Autodesk Inventor part; units mm, degrees
ref_plane "Start Plane" through (0, 0, -14.2929) normal (0, 0, 1) x (1, 0, 0)
ref_plane "End Plane" through (0, 0, 514.2929) normal (0, 0, 1) x (1, 0, 0)
ref_plane "Work Plane11" through (-7.7636, 7.7, -14.6464) normal (0.7071, 0, -0.7071) x (-0.7071, 0, -0.7071)
ref_plane "Start Plane" through (0, 0, -14.2929) normal (0, 0, 1) x (1, 0, 0)
ref_plane "End Plane" through (0, 0, 514.2929) normal (0, 0, 1) x (1, 0, 0)
sketch "Sketch" plane through (0, 0, 0) normal (0, 0, 1) x (1, 0, 0)
  line L0 (-2.41, 28.7) -> (-2.41, -7.3)
  line L1 (-7.41, 32.7) -> (-6.41, 32.7)
  line L2 (-7.41, -17.3) -> (-7.41, 32.7)
  line L3 (22.59, -17.3) -> (-7.41, -17.3)
  line L4 (22.59, -16.3) -> (22.59, -17.3)
  line L5 (2.59, -12.3) -> (18.59, -12.3)
  arc A0 (-2.41, -7.3) -> (2.59, -12.3) centre (2.59, -7.3) ccw
  arc A1 (-2.41, 28.7) -> (-6.41, 32.7) centre (-6.41, 28.7) ccw
  arc A2 (22.59, -16.3) -> (18.59, -12.3) centre (18.59, -16.3) ccw
  line L6 (0, 43.6941) -> (0, -27.4657) construction
  line L7 (-13.5757, 0) -> (29.5841, 0) construction
  point P0 (-2.41, 32.7)
  point P1 (-2.41, -12.3)
  point P2 (22.59, -12.3)
  dimension "d4" = 30
  dimension "d6" = 50
  dimension "d8" = 5
  dimension "d10" = 5
  dimension "d17" = 5
  dimension "d18" = 4
  dimension "d19" = 17.3
  dimension "d20" = 7.41
extrude "Body" add sketch "Sketch" along normal up to surface (528.5858 mm away) from surface at -14.2929
sketch "Sketch3" plane through (0, 0, 0) normal (0, 0, 1) x (1, 0, 0)
  line L0 (0, 0) -> (10, 0)
ref_plane "Work Plane10" through (0, 0, 0) normal (0, -1, 0) x (1, 0, 0)
sketch "Sketch4" plane through (0, 0, 0) normal (0, -1, 0) x (1, 0, 0)
  line L0 (-2, -14.2929) -> (12, -14.2929)
  line L1 (-2, 514.2929) -> (12, 514.2929)
  dimension "d24" = 528.5858
ref_plane "Work Plane11" through (-7.7636, 7.7, -14.6464) normal (0.7071, 0, -0.7071) x (-0.7071, 0, -0.7071)
split "Split1" plane through (-7.7636, 7.7, -14.6464) removes the side toward (0.7071, 0, -0.7071)
ref_plane "Work Plane12" through (-7.7636, 7.7, 514.6464) normal (0.7071, 0, 0.7071) x (0.7071, 0, -0.7071)
split "Split2" plane through (-7.7636, 7.7, 514.6464) removes the side toward (0.7071, 0, 0.7071)
equation "\"d4\" = b"
equation "\"d6\" = ParH"
equation "\"d17\" = R"
equation "\"d18\" = R1"
equation "\"d19\" = ex"
equation "\"d20\" = ey"
equation "\"d11\" = G_L"
equation "\"b\" = 30"
equation "\"ParT\" = 5"
equation "\"R1\" = 4"
equation "\"G_L\" = d24"
equation "\"ParH\" = 50"
equation "\"R\" = 5"
equation "\"ey\" = 7.41"
equation "\"ex\" = 17.3"
equation "\"G_OFFSET_START\" = 14.29289"
equation "\"G_OFFSET_END\" = 14.29289"
equation "\"d21\" = -G_OFFSET_START"
equation "\"d22\" = G_OFFSET_END + B_L"
properties part number "ISO 657-2 - 50x 30x 5-528.59" material "Steel, Mild"
The listing builds one solid part. Answer for the finished solid, in the listing's coordinates (mm). A direction names the side the tool comes from. Give positions to 0.01 mm unless a question says otherwise; leave off trailing zeros. Write each loop counter-clockwise with the first axis right and the second up, starting at its lowest first coordinate (ties: lowest second). Pieces come first, ordered by that corner, then holes. Notation, with made-up numbers: (-28.5, -40) - (26.5, -40) arc R27 cw to (26.5, -11) - close; hole circle Ø8 at (55.25, 3). An arc over 180 degrees is marked (long way). Use a Markdown table: item, result.
1. A tool of negligible diameter and unlimited length cuts with its end or side. For faces 1 (the flat face through (-3.59, 0.41, -10.47)), 2 (the flat face through (-2.41, 11, 246)), from which of +Z, -Z, +X, -X, +Y, -Y can it reach the whole face along a straight path? Write none if from no direction.
Values follow:
| item | result |
|---|---|
| face 1 | -Z, +X, +Y, -Y |
| face 2 | +Z, -Z, +X, +Y |
2. Section A-A on z = 256 is taken. Write down the section's boundary in (x, y).
Values follow:
| item | result |
|---|---|
| outline | (-7.41, -17.3) - (22.59, -17.3) - (22.59, -16.3) arc R4 ccw to (18.59, -12.3) - (2.59, -12.3) arc R5 cw to (-2.41, -7.3) - (-2.41, 28.7) arc R4 ccw to (-6.41, 32.7) - (-7.41, 32.7) - close |
3. Each of these flat-tipped pins is pushed along its axis until it touches: P1, Ø2, axis at x = -2.5, y = -3.5, coming from the -Z side; P2, Ø1, axis at x = 12.5, z = 163.5, coming from the +Y side. Where does it stop, or does it pass through?
Values follow:
| item | result |
|---|---|
| P1 | stops at z = -10.38 |
| P2 | stops at y = -12.3 |
4. Section B-B on y = 18 is taken. Write down the section's boundary in (x, z), plus the area to 3 significant figures.
Values follow:
| item | result |
|---|---|
| outline | (-7.41, -14.29) - (-2.41, -9.29) - (-2.41, 509.29) - (-7.41, 514.29) - close |
| area | 2,620 mm² |
5. Find the intervals of material crossed by probe 1 along Y at (x, z) = (-6, 60.5); probe 2 along Y at (x, z) = (13.5, 383); probe 3 along X at (y, z) = (20, 20.5), in increasing order. Write a range as from..to.
Values follow:
| item | result |
|---|---|
| probe 1 | y = -17.3..32.68 |
| probe 2 | y = -17.3..-12.3 |
| probe 3 | x = -7.41..-2.41 |
6. Section C-C on x = 10 is taken. Write down the section's boundary in (y, z), plus the area to 3 significant figures.
Values follow:
| item | result |
|---|---|
| outline | (-17.3, 3.12) - (-12.3, 3.12) - (-12.3, 496.88) - (-17.3, 496.88) - close |
| area | 2,470 mm² |
